Autodesk Inventor part; units mm, degrees
ref_plane "Arbeitsebene1" through (0, 15, 0) normal (0, 1, 0) x (-1, 0, 0)
ref_plane "YZ Plane" through (0, 0, 0) normal (1, 0, 0) x (0, 1, 0)
ref_plane "XY Plane" through (0, 0, 0) normal (0, 0, 1) x (1, 0, 0)
sketch "Skizze1" plane through (0, 0, 0) normal (0, 0, 1) x (1, 0, 0)
  line L0 (-56, 0) -> (56, 0)
  line L1 (0, -48.0323) -> (0, 183.1937)
  line L2 (40, 15) -> (40, -15)
  line L3 (40, -15) -> (-40, -15)
  line L4 (-40, -15) -> (-40, 15)
  arc A0 (-40, 15) -> (40, 15) centre (0, 150.1614) ccw
  point P0 (0, 0)
  dimension "d0" = 80
extrude "Extrusion1" add sketch "Skizze1" against normal blind 30
ref_plane "Arbeitsebene1" through (0, 15, 0) normal (0, 1, 0) x (-1, 0, 0)
sketch "Skizze3" plane through (0, 15, 0) normal (0, 1, 0) x (-1, 0, 0)
  line L0 (37.5, -2.5) -> (-37.5, -2.5)
  line L1 (-37.5, -2.5) -> (-37.5, -27.5)
  line L2 (-37.5, -27.5) -> (37.5, -27.5)
  line L3 (37.5, -27.5) -> (37.5, -2.5)
  line L4 (40, 0) -> (40, -30)
  line L5 (40, -30) -> (-40, -30)
  line L6 (-40, 0) -> (40, 0)
  line L7 (-40, 0) -> (-40, -30)
  point P0 (0, 0)
  dimension "d9" = 2.5
  dimension "d10" = 2.5
  dimension "d11" = 2.5
  dimension "d12" = 2.5
extrude "Extrusion2" cut sketch "Skizze3" against normal blind 27.5 contours L3 L2 L1 L0
sketch "Skizze4" plane through (-40, -15, 0) normal (0, -1, 0) x (1, 0, 0)
  line L0 (0, 0) -> (0, -30)
  line L1 (80, -30) -> (0, -30)
  point P0 (40, 0)
  point P1 (40, -15)
  dimension "d15" = 40
  dimension "d16" = 15
hole "Bohrung1" at (0, -15, -15) direction (0, 1, 0) diameter 9.3762 end through all
properties part number "Wasserablauf"
The listing builds one solid part. Answer for the finished solid, in the listing's coordinates (mm). A direction names the side the tool comes from. Give positions to 0.01 mm unless a question says otherwise; leave off trailing zeros. Write each loop counter-clockwise with the first axis right and the second up, starting at its lowest first coordinate (ties: lowest second). Pieces come first, ordered by that corner, then holes. Notation, with made-up numbers: (69, -38) -> (121, -38) arc R17 cw to (121, -16) -> close; hole circle Ø5 at (27.25, 75). An arc over 180 degrees is marked (long way). One line per question, with ' | ' between items. Start each with the question number.
1. Section C-C (y = 10) is taken. Determine the outline of the cut face in (x, z).
2. Given pin 1 Ø5 at (x, y) = (-26, -10.5) entering from +Z; pin 2 Ø1.5 at (x, z) = (5.5, -26.5) entering from +Y; pin 3 Ø5.5 at (x, z) = (0, -15) entering from -Y (3 decimals), each flat-ended and moving along its own axis, determine where each tip first touches the part or whether it passes through.
3. Section A-A (x = 0) is taken. Determine the outline of the cut face in (y, z), plus the area to 3 significant figures.
4. For faces 5 (the flat face through (37.5, 1, -15)), 6 (the cylindrical face through (-3.19, 9.24, -28.26)), determine the directions among +Z, -Z, +X, -X, +Y, -Y from which every point of the face is accessible in a straight line to the end or side of a thin tool.
5. Section D-D (z = -24.25) is taken. Determine the outline of the cut face in (x, y), plus the area to 3 significant figures.
6. Section B-B (z = -15) is taken. Determine the outline of the cut face in (x, y).
7. For a pull along Z with two mould halves and no side action, classify faces 1 (the flat face through (-40, 0, -15)), 2 (the flat face through (1, -2, -27.5)), 3 (the flat face through (-1, -3, 0)), 4 (the flat face through (-1, -3, -30)) as pulls with the +Z half, pulls with the -Z half, needs draft (parallel to the pull), parting line crosses it, or undercut.
8. Find the intervals of material crossed by probe 1 along Z at (x, y) = (0, -13.4); probe 2 along X at (y, z) = (13.5, -24.25); probe 3 along X at (y, z) = (-14.5, -15), in increasing order.
Response values:
1) outline: (-40, -30) -> (-14.95, -30) -> (-14.95, -27.5) -> (-37.5, -27.5) -> (-37.5, -2.5) -> (-14.95, -2.5) -> (-14.95, 0) -> (-40, 0) -> close; (14.95, -30) -> (40, -30) -> (40, 0) -> (14.95, 0) -> (14.95, -2.5) -> (37.5, -2.5) -> (37.5, -27.5) -> (14.95, -27.5) -> close
2) pin 1: z = 0 | pin 2: y = -12.5 | pin 3: through
3) outline: (-15, -30) -> (9.21, -30) -> (9.21, -27.5) -> (-12.5, -27.5) -> (-12.5, -19.69) -> (-15, -19.69) -> close; (-15, -10.31) -> (-12.5, -10.31) -> (-12.5, -2.5) -> (9.21, -2.5) -> (9.21, 0) -> (-15, 0) -> close | area: 160 mm2
4) face 5: +Y | face 6: +Z, -Z, +Y
5) outline: (-40, -15) -> (40, -15) -> (40, 15) arc R140.96 cw to (37.5, 14.29) -> (37.5, -12.5) -> (-37.5, -12.5) -> (-37.5, 14.29) arc R140.96 cw to (-40, 15) -> close | area: 336 mm2
6) outline: (-40, -15) -> (-4.69, -15) -> (-4.69, -12.5) -> (-37.5, -12.5) -> (-37.5, 14.29) arc R140.96 cw to (-40, 15) -> close; (4.69, -15) -> (40, -15) -> (40, 15) arc R140.96 cw to (37.5, 14.29) -> (37.5, -12.5) -> (4.69, -12.5) -> close
7) face 1: needs draft | face 2: undercut | face 3: pulls with the +Z half | face 4: pulls with the -Z half
8) probe 1: -30 to -19.69, -10.31 to 0 | probe 2: -40 to -37.5, 37.5 to 40 | probe 3: -40 to -4.69, 4.69 to 40
